```python
from build123d import *

# Parameters (mm, degrees)
SKETCH1_R               = 60
BOSS_EXTRUDE1_DEPTH     = 100
CUT_EXTRUDE1_DEPTH      = 452.895569028
CUT_EXTRUDE1_DEPTH_BACK = 452.895569028
SKETCH2_R               = 30
SKETCH9_R               = 60
CUT_EXTRUDE4_DEPTH      = 35
CUT_EXTRUDE5_DEPTH      = 457.59902747
SKETCH12_W              = 170
SKETCH12_H              = 275.29462827
CUT_EXTRUDE6_DEPTH      = 38.5


with BuildPart() as part:
    # Sketch1 → Boss-Extrude1 (new, symmetric)
    with BuildSketch(Plane.XY):
        with BuildLine():
            ThreePointArc((172.761636695, 269.924958208), (126.785478522, 271.892336111), (95.725474797, 305.847510456))
            Line((95.725474797, 305.847510456), (-20.619062469, 56.345845126))
            ThreePointArc((-20.619062469, 56.345845126), (25.357095704, 54.378467222), (56.417099429, 20.423292878))
            Line((56.417099429, 20.423292878), (172.761636695, 269.924958208))
        make_face()
        with Locations((152.142574227, 326.270803333)):
            Circle(SKETCH1_R)
        Circle(SKETCH1_R)
    extrude(amount=BOSS_EXTRUDE1_DEPTH, both=True)

    # Sketch2 → Cut-Extrude1 (cut, two sides: drawn at the far end of the back side and taken through both)
    with BuildSketch(Plane.XY.offset(-CUT_EXTRUDE1_DEPTH_BACK)):
        Circle(SKETCH2_R)
        with Locations((152.142574227, 326.270803333)):
            Circle(SKETCH2_R)
    extrude(amount=CUT_EXTRUDE1_DEPTH + CUT_EXTRUDE1_DEPTH_BACK, mode=Mode.SUBTRACT)

    # Sketch9 → Cut-Extrude4 (cut, symmetric)
    with BuildSketch(Plane.XY):
        with Locations((152.142574227, 326.270803333)):
            Circle(SKETCH9_R)
    extrude(amount=CUT_EXTRUDE4_DEPTH, both=True, mode=Mode.SUBTRACT)

    # Sketch10 → Cut-Extrude5 (cut, through all)
    with BuildSketch(Plane(origin=(-38.518080949, 17.961276124, 0), x_dir=(0, 0, 1), z_dir=(-0.906307787036651, 0.42261826174069733, 0))):
        with BuildLine():
            Line((-35, 317.647314135), (-35, 272.647314135))
            ThreePointArc((-35, 272.647314135), (-32.071067812, 265.576246323), (-25, 262.647314135))
            Line((-25, 262.647314135), (0, 262.647314135))
            Line((0, 262.647314135), (25, 262.647314135))
            ThreePointArc((25, 262.647314135), (32.071067812, 265.576246323), (35, 272.647314135))
            Line((35, 272.647314135), (35, 317.647314135))
            Line((35, 317.647314135), (-35, 317.647314135))
        make_face()
    extrude(amount=-CUT_EXTRUDE5_DEPTH, mode=Mode.SUBTRACT)

    # Sketch12 → Cut-Extrude6 (cut)
    with BuildSketch(Plane(origin=(-38.518080949, 17.961276124, 0), x_dir=(0, 0, 1), z_dir=(-0.906307787036651, 0.42261826174069733, 0))):
        with Locations((0, 180)):
            Rectangle(SKETCH12_W, SKETCH12_H)
    cut_extrude6 = extrude(amount=-CUT_EXTRUDE6_DEPTH, mode=Mode.SUBTRACT)

    # Mirror1: Cut-Extrude6 across plane
    add(cut_extrude6.mirror(Plane(origin=(0, 0, 0), x_dir=(0, 0, 1), z_dir=(-0.906307787036651, 0.42261826174069733, 0))), mode=Mode.SUBTRACT)


solid = part.part
```
Geometry check sheet. Reference: the model listing, model coordinates, mm. A direction names the side the tool comes from. Round coordinates to 2 decimals unless told otherwise and drop trailing zeros. Loops run counter-clockwise (first coordinate to the right, second up) from the corner with the lowest first, then second, coordinate; pieces in that order, holes last. Notation, with made-up numbers: (35.25, 37.5) - (39.25, 37.5) arc R18 ccw to (39.25, 50.5) - close; hole circle Ø9 at (78.5, -7.5). An arc over 180 degrees is marked (long way). Write item = value, one per line. Start each with the question number.
1. Section check C-C on x = 0. Enter the section's corners in (y, z), then the cut area to 3 significant figures.
2. Thickness scan on line 1 (Z direction, x = 170.5, y = 265.5); line 2 (X direction, y = 0, z = 11); line 3 (Y direction, x = 27.5, z = 2). Record the ranges inside material, lowest first.
3. Section check A-A on y = 0. Enter the section's corners in (x, z), then the cut area to 3 significant figures.
4. Mould release check, pull along Z, two halves, no side actions. Record for faces 1 (the face through (38.368, 182.843, -92.395)), 2 (the face through (75, 181, 100)), 3 (the face through (112.928, 297.826, 59.65)): released by +Z, released by -Z, zero draft, split by the parting line, or undercut.
5. Section check B-B on z = -20. Enter the section's corners in (x, y).
6. Set-up check for faces 4 (the face through (135, 354, 35)), 5 (the face through (39.215, 28.445, -1.19)), 6 (the face through (112.22, 240.79, -32.15)), 7 (the face through (-3.417, 48.324, -1.19)): record each of +Z, -Z, +X, -X, +Y, -Y from which the full face is reachable in a straight line by a thin tool's end or side.
7. Depth check by flat-ended pin: pin 1 (3 mm diameter, centred on x = 30, z = -19, fed in from +Y); pin 2 (1.5 mm diameter, centred on x = 25.5, z = -42, fed in from +Y); pin 3 (10 mm diameter, centred on x = 164, z = -29.5, fed in from +Y); pin 4 (3 mm diameter, centred on x = 50, z = -62, fed in from -Y). Enter the tip coordinate at first touch or a pass-through.
8. Section check D-D on y = 336. Enter the section's corners in (x, z), then the cut area to 3 significant figures.
Working result:
q1.outline = (-60, -100) - (-30, -100) - (-30, 100) - (-60, 100) - close; (30, -100) - (100.56, -100) - (100.56, -85) - (46.73, -85) - (46.73, 85) - (100.56, 85) - (100.56, 100) - (30, 100) - close
q1.area = 11,000 mm^2
q2.line_1 = -100 to -85, 85 to 100
q2.line_2 = -60 to -30, 30 to 60
q2.line_3 = -53.33 to -11.99, 11.99 to 33.91, 49.51 to 68.44
q3.outline = (-60, -100) - (-30, -100) - (-30, 100) - (-60, 100) - close; (30, -100) - (60, -100) - (60, 100) - (30, 100) - close
q3.area = 12,000 mm^2
q4.face_1 = zero draft
q4.face_2 = released by +Z
q4.face_3 = undercut
q5.outline = (-20.62, 56.35) arc R60 ccw (long way) to (56.42, 20.42) - (21.52, 36.69) - (114.62, 236.35) - (107.37, 239.73) - (14.27, 40.08) - close; hole circle Ø60 at (0, 0)
q6.face_4 = +X, -X, +Y
q6.face_5 = +X
q6.face_6 = +X, +Y
q6.face_7 = +Y
q7.pin_1 = 77.02
q7.pin_2 = 65.76
q7.pin_3 = through
q7.pin_4 = -35.32
q8.outline = (92.94, -100) - (123.76, -100) - (123.76, -35) - (92.94, -35) - close; (92.94, 35) - (123.76, 35) - (123.76, 100) - (92.94, 100) - close; (180.52, -100) - (211.35, -100) - (211.35, -35) - (180.52, -35) - close; (180.52, 35) - (211.35, 35) - (211.35, 100) - (180.52, 100) - close
q8.area = 8,020 mm^2
